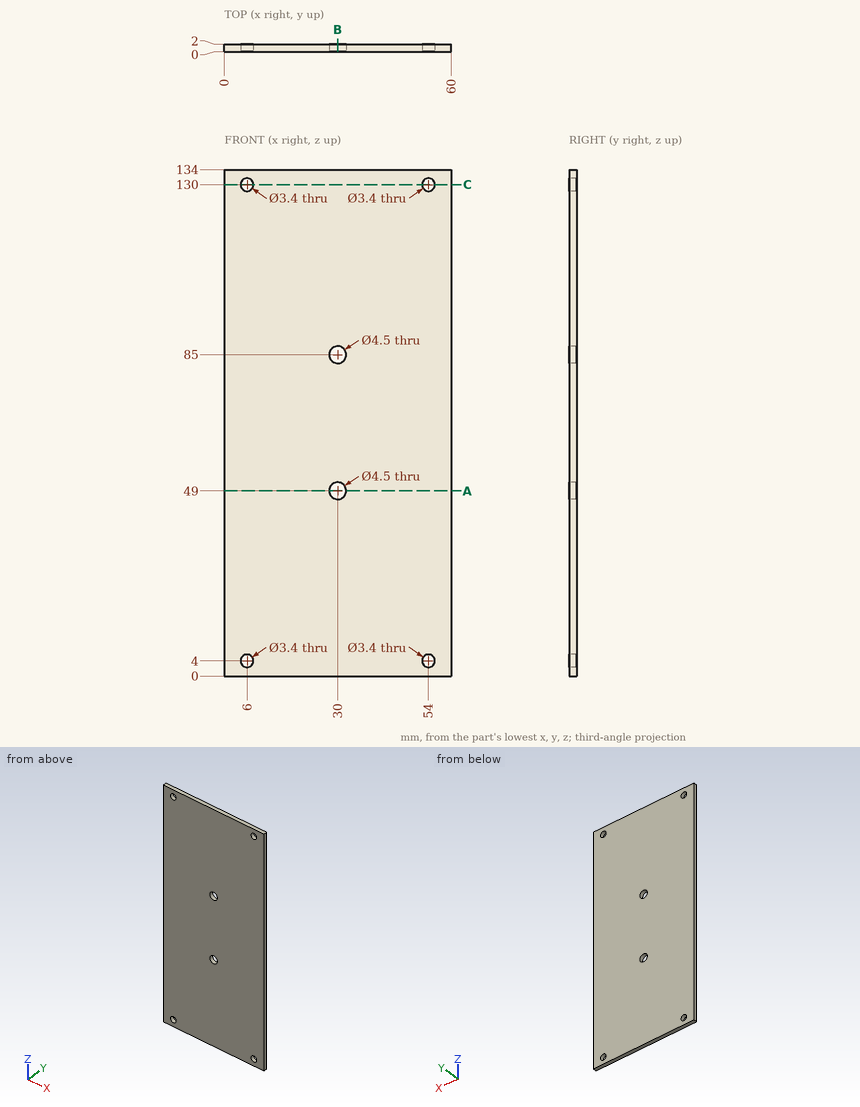
The figure shows three views and two pictorial views of one solid part (mm, origin at its lowest corner). Answer the questions. Coordinates: 2 decimals unless noted, no trailing zeros. Order: outer loops, then holes, each group sorted by start corner. A loop starts at its lowest first (then second) coordinate and runs counter-clockwise, first axis right, second up. Notation, with made-up numbers: M 68,86 L 126,86 A12 cw 126,95 Z; hole C 4,80 d7. An arc over 180 degrees is marked long. Use CSV: the item, a comma, the result in double quotes.
1) Section C-C on z = 130 is taken. Write down the section's boundary in (x, y), plus the area to 3 significant figures.
Worked out:
outline,"M 0,0 L 4.3,0 L 4.3,2 L 0,2 Z; M 7.7,0 L 52.3,0 L 52.3,2 L 7.7,2 Z; M 55.7,0 L 60,0 L 60,2 L 55.7,2 Z"
area,"106 mm^2"
2) A flat-ended cylindrical pin translates along its axis: pin 1 Ø1 at (y, z) = (1.5, 97.5) entering from -X. Find the tip coordinate at first contact, or state that the pin passes through.
Worked out:
pin 1,"stops at x = 0"
3) Section A-A on z = 49 is taken. Write down the section's boundary in (x, y).
Worked out:
outline,"M 0,0 L 27.75,0 L 27.75,2 L 0,2 Z; M 32.25,0 L 60,0 L 60,2 L 32.25,2 Z"
4) Section B-B on x = 30 is taken. Write down the section's boundary in (y, z).
Worked out:
outline,"M 0,0 L 2,0 L 2,46.75 L 0,46.75 Z; M 0,51.25 L 2,51.25 L 2,82.75 L 0,82.75 Z; M 0,87.25 L 2,87.25 L 2,134 L 0,134 Z"
5) Consider line 1 (Z direction, x = 30, y = 1.5); line 2 (Z direction, x = 54, y = 0.7); line 3 (X direction, y = 1.15, z = 130). Determine where each line is inside the solid, lowest interval first. Write a range as [from, to].
Worked out:
line 1,"z = [0, 46.75], [51.25, 82.75], [87.25, 134]"
line 2,"z = [0, 2.3], [5.7, 128.3], [131.7, 134]"
line 3,"x = [0, 4.3], [7.7, 52.3], [55.7, 60]"
